Here's how the part is built. I have some questions about the finished solid (model axes, mm). A direction names the side the tool comes from. Give positions to 0.01 mm unless a question says otherwise; leave off trailing zeros. Loops run counter-clockwise (first coordinate to the right, second up) from the corner with the lowest first, then second, coordinate; pieces in that order, holes last. Notation, with made-up numbers: M 11,10.25 L 63,10.25 A21 ccw 63,44.25 Z; hole C 48,66 d7. An arc over 180 degrees is marked long. Answer as CSV lines item,"result". Start each with the question number.
Item 1: If we mould it in two halves opening along Z, with no side actions, what happens to faces 4 (the cylindrical face through (-4.769, 55.431, 21.477)), 5 (the cylindrical face through (60.967, 6.444, 25.278)), 6 (the cylindrical face through (48.58, 1.48, -50.4))? For each: released by +Z, released by -Z, zero draft, split by the parting line, or undercut.
Item 2: I want a section at B-B on y = 18.5. List the corners of the cut face in (x, z) for me, plus the area to 3 significant figures.
Item 3: Will these pins go through, and if not, where does the flat tip stop? P1, Ø2, axis at y = 55, z = -7, coming from the +X side; P2, Ø2.5, axis at x = 73, y = 2, coming from the -Z side; P3, Ø1.5, axis at x = 46, y = 2, coming from the +Z side.
Item 4: For faces 1 (the cylindrical face through (29.07, 3.91, 55.89)), 2 (the flat face through (55.4, 3, 40.1)), 3 (the flat face through (1.7, 63, 22.1)), which set-ups out of +Z, -Z, +X, -X, +Y, -Y let a thin tool reach every point of the face, with its end or its side?
Item 5: I want a section at A-A on y = 52.5. List the corners of the cut face in (x, z) for me, plus the area to 3 significant figures.
Item 6: If I drill on line 1 along X through (y, z) = (59.25, 0); line 2 along Z through (x, y) = (84.93, 2.45); line 3 along X through (y, z) = (3.25, 0), over which ranges is the centre line in solid material (lowest first)? Write a range as from..to.
from build123d import *

# Parameters (mm, degrees)
SKETCH2_R           = 63
BOSS_EXTRUDE1_DEPTH = 3
SKETCH3_R           = 66
SKETCH3_R_2         = 63
BOSS_EXTRUDE2_DEPTH = 10
SKETCH7_R           = 25
SKETCH7_R_2         = 22
BOSS_EXTRUDE3_DEPTH = 20
FILLET1_R           = 10
FILLET2_R           = 2
SKETCH8_W           = 8
SKETCH8_H           = 8
SKETCH8_R           = 1.75
BOSS_EXTRUDE4_DEPTH = 3
FILLET3_R           = 3
SKETCH9_R           = 1.75
CUT_EXTRUDE1_DEPTH  = 4.0000001


with BuildPart() as part:
    # Sketch2 → Boss-Extrude1 (new body)
    with BuildSketch(Plane(origin=(0, 0, 0), x_dir=(1, 0, 0), z_dir=(0, 1, 0))):
        with BuildLine():
            Line((0, -70), (90, -70))
            Line((90, -70), (90, 0))
            Line((90, 0), (70, 0))
            ThreePointArc((70, 0), (-49.497474683, 49.497474683), (0, -70))
        make_face()
        Circle(SKETCH2_R, mode=Mode.SUBTRACT)
    extrude(amount=BOSS_EXTRUDE1_DEPTH)

    # Sketch3 → Boss-Extrude2 (add)
    with BuildSketch(Plane(origin=(0, 3, 0), x_dir=(1, 0, 0), z_dir=(0, 1, 0))):
        Circle(SKETCH3_R)
        Circle(SKETCH3_R_2, mode=Mode.SUBTRACT)
    extrude(amount=BOSS_EXTRUDE2_DEPTH)

    # Sketch6 → Revolve1 (revolve)
    with BuildSketch(Plane(origin=(0, 0, 0), x_dir=(0, 0, -1), z_dir=(1, 0, 0))):
        Polygon((-66, 13), (-25, 43), (-22, 43), (-63, 13), align=None)
    revolve(axis=Axis((0, 0, 0), (0, 1, 0)))

    # Sketch7 → Boss-Extrude3 (add)
    with BuildSketch(Plane(origin=(0, 43, 0), x_dir=(1, 0, 0), z_dir=(0, 1, 0))):
        Circle(SKETCH7_R)
        Circle(SKETCH7_R_2, mode=Mode.SUBTRACT)
    extrude(amount=BOSS_EXTRUDE3_DEPTH)

    # Fillet1
    fillet1_edges = [part.edges().sort_by_distance(p)[0] for p in [
        (46.669047558, 13, 46.669047558),
        (-15.556349186, 43, -15.556349186),
        (-44.547727215, 13, -44.547727215),
        (17.67766953, 43, 17.67766953),
    ]]
    fillet(fillet1_edges, radius=FILLET1_R)

    # Fillet2
    fillet2_edges = [part.edges().sort_by_distance(p)[0] for p in [
        (-66, 3, 0),
    ]]
    fillet(fillet2_edges, radius=FILLET2_R)

    # Sketch8 → Boss-Extrude4 (add)
    with BuildSketch(Plane.XZ):
        with Locations((73.541354603, -4)):
            Rectangle(SKETCH8_W, SKETCH8_H)
        with Locations((73.541354603, -4)):
            Circle(SKETCH8_R, mode=Mode.SUBTRACT)
        with Locations((73.541354603, 74)):
            Rectangle(SKETCH8_W, SKETCH8_H)
        with Locations((73.541354603, 74)):
            Circle(SKETCH8_R, mode=Mode.SUBTRACT)
        with Locations((-73.885620839, 0)):
            Rectangle(SKETCH8_W, SKETCH8_H)
        with Locations((-73.885620839, 0)):
            Circle(SKETCH8_R, mode=Mode.SUBTRACT)
        with Locations((0, -73.885620839)):
            Rectangle(SKETCH8_W, SKETCH8_H)
        with Locations((0, -73.885620839)):
            Circle(SKETCH8_R, mode=Mode.SUBTRACT)
        with Locations((4, 74)):
            Rectangle(SKETCH8_W, SKETCH8_H)
        with Locations((4, 74)):
            Circle(SKETCH8_R, mode=Mode.SUBTRACT)
    extrude(amount=-BOSS_EXTRUDE4_DEPTH)

    # Fillet3
    fillet3_edges = [part.edges().sort_by_distance(p)[0] for p in [
        (-4, 1.5, -77.885620839),
        (-4, 1.5, -69.885620839),
        (4, 1.5, -69.885620839),
        (4, 1.5, -77.885620839),
        (0, 1.5, 78),
        (8, 1.5, 78),
        (8, 1.5, 70),
        (77.541354603, 1.5, 0),
        (77.541354603, 1.5, -8),
        (69.541354603, 1.5, -8),
        (77.541354603, 1.5, 78),
        (77.541354603, 1.5, 70),
        (69.541354603, 1.5, 70),
        (69.541354603, 1.5, 78),
        (0, 1.5, 70),
        (-69.885620839, 1.5, 4),
        (-69.885620839, 1.5, -4),
        (-77.885620839, 1.5, -4),
        (-77.885620839, 1.5, 4),
    ]]
    fillet(fillet3_edges, radius=FILLET3_R)

    # Sketch9 → Cut-Extrude1 (cut, through all)
    with BuildSketch(Plane(origin=(0, 3, 0), x_dir=(1, 0, 0), z_dir=(0, 1, 0))):
        with Locations((84.93, -10)):
            Circle(SKETCH9_R)
        with Locations((84.93, -60)):
            Circle(SKETCH9_R)
    extrude(amount=-CUT_EXTRUDE1_DEPTH, mode=Mode.SUBTRACT)


solid = part.part
Result:
1,face 4,"undercut"
1,face 5,"split by the parting line"
1,face 6,"released by -Z"
2,outline,"C 0,0 d116.97; hole C 0,0 d110.97"
2,area,"1,070 mm^2"
3,P1,"x = 24.27"
3,P2,"z = -8.03"
3,P3,"z = 70"
4,face 1,"-Y"
4,face 2,"+Y"
4,face 3,"+Z, -Z, +X, -X, +Y"
5,outline,"C 0,0 d50; hole C 0,0 d44"
5,area,"443 mm^2"
6,line 1,"-25..-22, 22..25"
6,line 2,"0..8.25, 11.75..58.25, 61.75..70"
6,line 3,"-67.03..-63, 63..67.03"
